Read the model definition and answer for the solid it produces. Units are mm, in the model's axes. A direction names the side the tool comes from. Coordinates: 2 decimals unless noted, no trailing zeros. Loops run counter-clockwise (first coordinate to the right, second up) from the corner with the lowest first, then second, coordinate; pieces in that order, holes last. Notation, with made-up numbers: (-34.5, -6.5) - (-4.5, -6.5) arc R12 ccw to (-4.5, 15.5) - close; hole circle Ø7 at (8.25, -39.5). An arc over 180 degrees is marked (long way). Use one line per item in the form item = value. Start each with the question number.
1) Each of these flat-tipped pins is pushed along its axis until it touches: P1, Ø5, axis at x = 3, z = 10.5, coming from the +Y side; P2, Ø1.5, axis at x = 3, y = -3, coming from the +Z side; P3, Ø1.5, axis at x = -3, z = 5, coming from the +Y side; P4, Ø2.5, axis at x = 0.5, y = -1, coming from the -Z side. Where does it stop, or does it pass through?
2) Which of the six approach directions +Z, -Z, +X, -X, +Y, -Y give full straight-line access (tool end or side, diameter ignored) to faces 1 (the face through (2, -2, 8.89)), 2 (the face through (-1.27, 0, 11))?
3) The mould has two halves that part along X. Classify faces 3 (the face through (0, 3.175, 11)), 4 (the face through (0, 0, 0)), 5 (the face through (-0.33, 2.52, 4.38)): released by +X, released by -X, zero draft, split by the parting line, or undercut.
4) Consider line 1 (Z direction, x = 1, y = 1.75); line 2 (X direction, y = -1, z = 10.25); line 3 (Z direction, x = -1.75, y = -1). Determine where each line is inside the solid, lowest interval first.
5) A cutting plane is placed at A-A (z = 5.5). Give the vertices of the cut face in (x, y).
from build123d import *

# Parameters (mm, degrees)
F0_R     = 2.54
F1_DEPTH = 8.89
F2_R     = 4.445
F3_DEPTH = 3.81
F4_W     = 2.54
F4_H     = 6.35
F5_DEPTH = 2.54


# Not quite as in the source:
# - a fillet or chamfer that OpenCascade refuses, or shapes differently, is made with other operations: its cross-section is extruded or revolved along the edge and cut away or added


with BuildPart() as f1:
    # F0 (on Top) → F1 (new body)
    with BuildSketch(Plane.XY):
        Circle(F0_R)
    extrude(amount=F1_DEPTH)

    # F2 (on face) → F3 (join)
    with BuildSketch(Plane.XY.offset(8.89)):
        Circle(F2_R)
    extrude(amount=F3_DEPTH)

    # F4 (on face) → F5 (cut)
    with BuildSketch(Plane.XY.offset(12.7)):
        Rectangle(F4_W, F4_H)
    extrude(amount=-F5_DEPTH, mode=Mode.SUBTRACT)

    # F6: fillet of radius 3.81 on 1 edges, made by hand

    # F6_s1 → F6_t2 (revolve, cut)
    with BuildSketch(Plane.XZ):
        with BuildLine():
            ThreePointArc((4.445, 8.89), (3.3290768363, 11.5840768363), (0.635, 12.7))
            Line((0.635, 12.7), (4.445, 12.7))
            Line((4.445, 12.7), (4.445, 8.89))
        make_face()
    revolve(axis=Axis((0, 0, 12.7), (0, 0, 1)), mode=Mode.SUBTRACT)


solid = f1.part
Found:
q1.P1 = 4.35
q1.P2 = 11.41
q1.P3 = 1.18
q1.P4 = 0
q2.face_1 = -Z
q2.face_2 = +Z
q3.face_3 = undercut
q3.face_4 = zero draft
q3.face_5 = split by the parting line
q4.line_1 = 0 to 10.16
q4.line_2 = -4.07 to -1.27, 1.27 to 4.07
q4.line_3 = 0 to 12.44
q5.outline = circle Ø5.08 at (0, 0)
